Can you work these out from the model? Positions are in its coordinate system, mm. A direction names the side the tool comes from. Coordinates: 2 decimals unless noted, no trailing zeros. Order: outer loops, then holes, each group sorted by start corner. A loop starts at its lowest first (then second) coordinate and runs counter-clockwise, first axis right, second up. Notation, with made-up numbers: (-31, 28.25) - (1, 28.25) arc R30 cw to (1, 59.25) - close; hole circle Ø9 at (34, 38). An arc over 180 degrees is marked (long way). Use a Markdown table: item, result. Add a question column.
(1) On a 3-axis mill with a long thin cutter (end or side, diameter ignored), from which of +Z, -Z, +X, -X, +Y, -Y can I reach the whole of each face in a straight line? I mean faces 4 (the flat face through (11.8, 493, 0)), 5 (the flat face through (-12.8, 493, 0)). Say none if no direction works.
(2) I want a section at B-B (z = 0.5). List the corners of the cut face in (x, y) for me.
(3) We'd pull the mould along X, two halves only. Please class faces 1 (the flat face through (0, 493, -12.8)), 2 (the flat face through (-11.8, 493, 0)), 3 (the flat face through (12.8, 493, 0)): pulls with the +X half, pulls with the -X half, needs draft (parallel to the pull), parting line crosses it, or undercut.
(4) If I drill on L1, parallel to X at y = 217.2, z = 12.4; L2, parallel to X at y = 873.5, z = 3.25, over which ranges is the centre line in solid material (lowest first)? Write a range as [from, to].
(5) I want a section at C-C (y = 70). List the corners of the cut face in (x, z) for me, and give its area (3 significant figures).
(6) I want a section at A-A (x = -7.25). List the corners of the cut face in (y, z) for me, and give its area (3 significant figures).
```python
from build123d import *

# Parameters (mm, degrees)
SKETCH1_W           = 25.6
SKETCH1_H           = 25.6
SKETCH1_W_2         = 23.6
SKETCH1_H_2         = 23.6
BOSS_EXTRUDE1_DEPTH = 1000
SKETCH2_R           = 2
CUT_EXTRUDE1_DEPTH  = 33


with BuildPart() as part:
    # Sketch1 → Boss-Extrude1 (new body)
    with BuildSketch(Plane(origin=(0, 0, 0), x_dir=(1, 0, 0), z_dir=(0, 1, 0))):
        Rectangle(SKETCH1_W, SKETCH1_H)
        Rectangle(SKETCH1_W_2, SKETCH1_H_2, mode=Mode.SUBTRACT)
    extrude(amount=BOSS_EXTRUDE1_DEPTH)

    # Sketch2 → Cut-Extrude1 (cut)
    with BuildSketch(Plane(origin=(0, 0, -12.8), x_dir=(-1, 0, 0), z_dir=(0, 0, -1))):
        with Locations((0, 535)):
            Circle(SKETCH2_R)
        with Locations((0, 465)):
            Circle(SKETCH2_R)
        with Locations((0, 782.8)):
            Circle(SKETCH2_R)
        with Locations((0, 712.8)):
            Circle(SKETCH2_R)
        with Locations(Location((0, 287.2, 0), (0, 0, 180))):
            Circle(SKETCH2_R)
        with Locations(Location((0, 217.2, 0), (0, 0, 180))):
            Circle(SKETCH2_R)
    extrude(amount=-CUT_EXTRUDE1_DEPTH, mode=Mode.SUBTRACT)


solid = part.part
```
Answers follow:
| question | item | result |
|---|---|---|
| 1 | face 4 | +Y, -Y |
| 1 | face 5 | +Z, -Z, -X, +Y, -Y |
| 2 | outline | (-12.8, 0) - (-11.8, 0) - (-11.8, 1000) - (-12.8, 1000) - close; (11.8, 0) - (12.8, 0) - (12.8, 1000) - (11.8, 1000) - close |
| 3 | face 1 | needs draft |
| 3 | face 2 | undercut |
| 3 | face 3 | pulls with the +X half |
| 4 | L1 | x = [-12.8, -2], [2, 12.8] |
| 4 | L2 | x = [-12.8, -11.8], [11.8, 12.8] |
| 5 | outline | (-12.8, -12.8) - (12.8, -12.8) - (12.8, 12.8) - (-12.8, 12.8) - close; hole (-11.8, -11.8) - (11.8, -11.8) - (11.8, 11.8) - (-11.8, 11.8) - close |
| 5 | area | 98.4 mm² |
| 6 | outline | (0, -12.8) - (1000, -12.8) - (1000, -11.8) - (0, -11.8) - close; (0, 11.8) - (1000, 11.8) - (1000, 12.8) - (0, 12.8) - close |
| 6 | area | 2,000 mm² |
